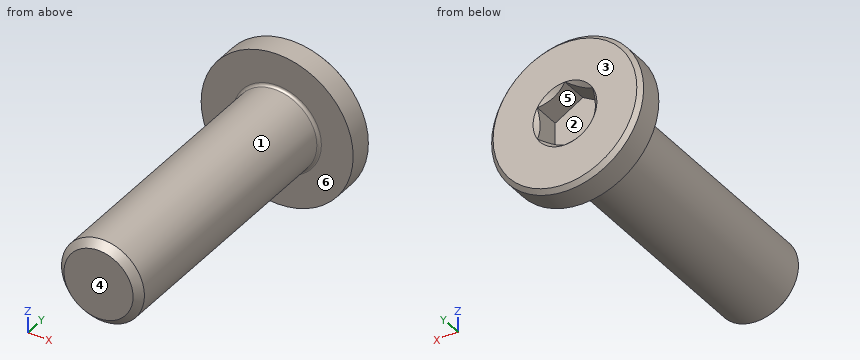
Autodesk Inventor part; units mm, degrees
ref_plane "YZ Plane" through (0, 0, 0) normal (1, 0, 0) x (0, 1, 0)
ref_plane "XZ Plane" through (0, 0, 0) normal (0, 1, 0) x (-1, 0, 0)
ref_plane "XY Plane" through (0, 0, 0) normal (0, 0, 1) x (1, 0, 0)
sketch "Sketch1" plane through (0, 0, 0) normal (0, 0, 1) x (1, 0, 0)
  line L0 (0, 5.5) -> (0, -5.5)
  line L1 (0, -5.5) -> (1.25, -5.5)
  line L2 (1.25, -5.5) -> (1.5, -5.25)
  line L3 (1.5, -5.25) -> (1.5, 4.4)
  line L4 (1.6, 4.5) -> (2.75, 4.5)
  line L5 (2.75, 4.5) -> (2.75, 5.35)
  line L6 (2.6, 5.5) -> (0, 5.5)
  arc A0 (1.6, 4.5) -> (1.5, 4.4) centre (1.6, 4.4) ccw
  line L7 (2.6, 5.5) -> (2.75, 5.35)
  point P0 (0, 0)
  point P1 (2.75, 5.5)
  point P2 (0, 0)
  dimension "d0" = 5.5
  dimension "d1" = 1
  dimension "d3" = 3
  dimension "d4" = 3.2
  dimension "d5" = 135
  dimension "d6" = 0.25
  dimension "d7" = 10
  dimension "d18" = 0.15
  dimension "d22" = 0.15
revolve "Revolution1" add sketch "Sketch1" angle 360 about axis through (0, 5.5, 0) along (0, -1, 0)
sketch "Sketch2" plane through (0, 5.5, 0) normal (0, 1, 0) x (1, 0, 0)
  line L0 (0, -1.1547) -> (-1, -0.5774)
  line L1 (-1, -0.5774) -> (-1, 0.5774)
  line L2 (-1, 0.5774) -> (0, 1.1547)
  line L3 (0, 1.1547) -> (1, 0.5774)
  line L4 (1, 0.5774) -> (1, -0.5774)
  line L5 (1, -0.5774) -> (0, -1.1547)
  point P0 (0, 0)
  point P1 (0, 0)
  dimension "d11" = 2
extrude "Extrusion1" cut sketch "Sketch2" against normal blind 1
thread "Thread1"
sketch "Sketch3" plane through (0, 0, 0) normal (1, 0, 0) x (0, 1, 0)
  line L0 (5.5, 1.1547) -> (5.5, 0.5774)
  line L1 (5.5, 1.1547) -> (5, 0.6547)
  line L2 (5, 0.6547) -> (5.5, 0.6547)
  line L3 (5.5, 0.6547) -> (5.5, 1.1547)
  line L4 (-0.9, 0) -> (5.4, 0)
  point P0 (0, 0)
  dimension "d16" = 0.5
revolve "Revolution2" cut sketch "Sketch3" angle 360 about axis through (0, -10, 0) along (0, 1, 0)
equation "\"d22\" = d18"
properties part number "48-03A1" material "Stainless Steel"
Geometry check sheet. Reference: the model listing, model coordinates, mm. Face numbers are marked on the shaded views. A direction names the side the tool comes from. Round coordinates to 2 decimals unless told otherwise and drop trailing zeros. Loops run counter-clockwise (first coordinate to the right, second up) from the corner with the lowest first, then second, coordinate; pieces in that order, holes last. Notation, with made-up numbers: (20, 56) - (74, 56) arc R19 ccw to (74, 72) - close; hole circle Ø11 at (-21, -23.5). An arc over 180 degrees is marked (long way). One line per question, with ' | ' between items. Start each with the question number.
1. Depth check by flat-ended pin: pin 1 (1.6 mm diameter, centred on x = 0.5, z = 0.5, fed in from +Y); pin 2 (2 mm diameter, centred on y = 2, z = 1.5, fed in from +X). Enter the tip coordinate at first touch or a pass-through.
2. Scan lines: line 1 (Y direction, x = -2.35, z = 0.5); line 2 (X direction, y = -2.25, z = -0.05); line 3 (X direction, y = 5.25, z = -0.5). Record each from-to range of solid material in increasing order. Write a range as [from, to].
3. Cross-section at B-B on y = -2.5. Record the cut outline in (x, z), then the cut area to 3 significant figures.
4. Cross-section at A-A on z = 0. Record the cut outline in (x, y), then the cut area to 3 significant figures.
5. Tool access check on the marked faces 4, 5 and 6. Record the directions out of +Z, -Z, +X, -X, +Y, -Y that give a thin tool (end or side, any length) a straight path to the whole face; none if there is none.
6. Draft check along Z on the marked faces 1, 2 and 3. Enter one of: released by +Z, released by -Z, zero draft, split by the parting line, or undercut.
Taken from the geometry:
1) pin 1: y = 5.5 | pin 2: x = 1.41
2) line 1: [4.5, 5.5] | line 2: [-1.5, 1.5] | line 3: [-2.7, -1], [1, 2.7]
3) outline: circle Ø3 at (0, 0) | area: 7.07 mm²
4) outline: (-2.75, 4.5) - (-1.6, 4.5) arc R0.1 cw to (-1.5, 4.4) - (-1.5, -5.25) - (-1.25, -5.5) - (1.25, -5.5) - (1.5, -5.25) - (1.5, 4.4) arc R0.1 cw to (1.6, 4.5) - (2.75, 4.5) - (2.75, 5.35) - (2.6, 5.5) - (1.15, 5.5) - (1, 5.35) - (1, 4.5) - (-1, 4.5) - (-1, 5.35) - (-1.15, 5.5) - (-2.6, 5.5) - (-2.75, 5.35) - close | area: 33.4 mm²
5) face 4: +Z, -Z, +X, -X, -Y | face 5: +Y | face 6: -Y
6) face 1: split by the parting line | face 2: undercut | face 3: zero draft
